```python
from build123d import *

# Parameters (mm, degrees)
SKETCH1_W               = 360
SKETCH1_H               = 540
BOSS_EXTRUDE1_DEPTH     = 3
CUT_EXTRUDE1_DEPTH      = 325.513482
CUT_EXTRUDE1_DEPTH_BACK = 325.513482
SKETCH2_R               = 5


with BuildPart() as part:
    # Sketch1 → Boss-Extrude1 (new body)
    with BuildSketch(Plane(origin=(0, 0, 0), x_dir=(1, 0, 0), z_dir=(0, 1, 0))):
        Rectangle(SKETCH1_W, SKETCH1_H)
    extrude(amount=BOSS_EXTRUDE1_DEPTH)

    # Sketch2 → Cut-Extrude1 (cut, two sides: drawn at the far end of the back side and taken through both)
    with BuildSketch(Plane(origin=(0, 3, 0), x_dir=(1, 0, 0), z_dir=(0, 1, 0)).offset(-CUT_EXTRUDE1_DEPTH_BACK)):
        with Locations(Location((-167.5, 212.5, 0), (0, 0, 270))):
            Circle(SKETCH2_R)
        with Locations(Location((-167.5, 165, 0), (0, 0, 270))):
            Circle(SKETCH2_R)
        with Locations(Location((-167.5, 260, 0), (0, 0, 90))):
            Circle(SKETCH2_R)
        with Locations(Location((167.5, 260, 0), (0, 0, 270))):
            Circle(SKETCH2_R)
        with Locations(Location((167.5, 165, 0), (0, 0, 90))):
            Circle(SKETCH2_R)
        with Locations(Location((167.5, 212.5, 0), (0, 0, 90))):
            Circle(SKETCH2_R)
    extrude(amount=CUT_EXTRUDE1_DEPTH + CUT_EXTRUDE1_DEPTH_BACK, mode=Mode.SUBTRACT)


solid = part.part
```
Input: part model. Units: mm. Frame: model coordinates. Give positions to 0.01 mm unless a question says otherwise; leave off trailing zeros.
1. Draft query along Z for faces 1 (the face through (-3, 0, -4)), 2 (the face through (-166, 1.48, -207.73)). Return one class per face: released by +Z, released by -Z, zero draft, split by the parting line, or undercut.
Computed:
face 1: zero draft
face 2: undercut
2. Pin query (flat end, axial travel): pin 1 Ø6 at (x, z) = (167.5, -212.5) entering from -Y. Return the tip coordinate at first contact, or that it passes through.
Computed:
pin 1: passes through
3. Line query: probe 1 along X at (y, z) = (1.6, -212.5); probe 2 along Z at (x, y) = (-164, 1.6). Output: solid intervals per line, ascending.
Computed:
probe 1: x = -180 to -172.5, -162.5 to 162.5, 172.5 to 180
probe 2: z = -270 to -263.57, -256.43 to -216.07, -208.93 to -168.57, -161.43 to 270
